```python
from build123d import *

# Parameters (mm, degrees)
BOSS_EXTRUDE1_DEPTH     = 10
CUT_EXTRUDE1_DEPTH      = 47.432747065
CUT_EXTRUDE1_DEPTH_BACK = 47.432747065
SKETCH2_R               = 1.65
CHAMFER1_SIZE           = 1.6
FILLET1_R               = 3
FILLET3_R               = 5


with BuildPart() as part:
    # Sketch1 → Boss-Extrude1 (new body)
    with BuildSketch(Plane.XY):
        Polygon((0, 0), (0, 5), (-13, 5), (-13, 25), (0, 25), (0, 30), (-34, 30), (-34, 25), (-21, 25), (-21, 5), (-34, 5), (-34, 0), align=None)
    extrude(amount=BOSS_EXTRUDE1_DEPTH)

    # Sketch2 → Cut-Extrude1 (cut, two sides: drawn at the far end of the back side and taken through both)
    with BuildSketch(Plane(origin=(0, 30, 0), x_dir=(1, 0, 0), z_dir=(0, 1, 0)).offset(-CUT_EXTRUDE1_DEPTH_BACK)):
        with Locations(Location((-30, -5, 0), (0, 0, 180))):
            Circle(SKETCH2_R)
        with Locations(Location((-4, -5, 0), (0, 0, 180))):
            Circle(SKETCH2_R)
    extrude(amount=CUT_EXTRUDE1_DEPTH + CUT_EXTRUDE1_DEPTH_BACK, mode=Mode.SUBTRACT)

    # Chamfer1
    chamfer1_edges = [part.edges().sort_by_distance(p)[0] for p in [
        (-28.35, 5, 5),
        (-2.35, 5, 5),
    ]]
    chamfer(chamfer1_edges, length=CHAMFER1_SIZE)

    # Fillet1
    fillet1_edges = [part.edges().sort_by_distance(p)[0] for p in [
        (-21, 5, 5),
        (-21, 25, 5),
        (-13, 25, 5),
        (-13, 5, 5),
    ]]
    fillet(fillet1_edges, radius=FILLET1_R)

    # Fillet3
    fillet3_edges = [part.edges().sort_by_distance(p)[0] for p in [
        (-34, 2.5, 0),
        (-34, 2.5, 10),
        (0, 2.5, 10),
        (0, 2.5, 0),
        (0, 27.5, 0),
        (0, 27.5, 10),
        (-34, 27.5, 0),
        (-34, 27.5, 10),
    ]]
    fillet(fillet3_edges, radius=FILLET3_R - 0.0001)  # a hair under: the kernel refuses the full size


solid = part.part
```
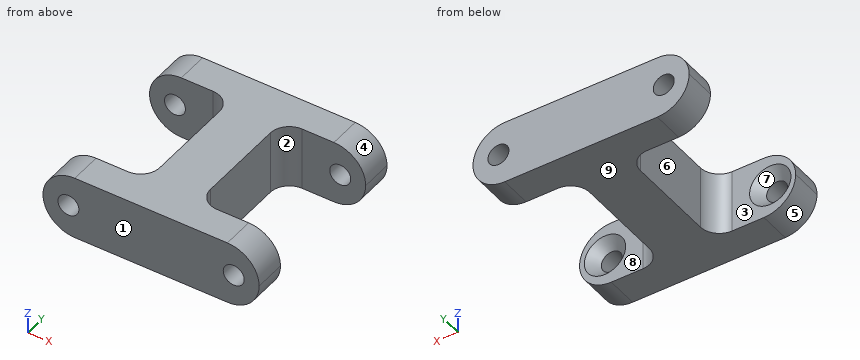
Geometry check sheet. Reference: the model listing, model coordinates, mm. Face numbers are marked on the shaded views. A direction names the side the tool comes from. Coordinates: 2 decimals unless noted, no trailing zeros. Order: outer loops, then holes, each group sorted by start corner. A loop starts at its lowest first (then second) coordinate and runs counter-clockwise, first axis right, second up. Notation, with made-up numbers: (-35.5, 88) - (8.5, 88) arc R26 cw to (8.5, 127) - close; hole circle Ø9 at (29, 89.5). An arc over 180 degrees is marked (long way). Answer as a JSON object with one key per item and string values. Group by question number.
Item 1: Sectioned sample at A-A, the plane x = -11.5. Record the cut outline in (y, z).
Item 2: Depth check by flat-ended pin: pin 1 Ø3 at (y, z) = (8, 2) entering from +X; pin 2 Ø6 at (y, z) = (11.5, 4) entering from +X; pin 3 Ø3 at (y, z) = (14, 6) entering from -X. Enter the tip coordinate at first touch or a pass-through.
Item 3: Sectioned sample at C-C, the plane z = 8.75. Record the cut outline in (x, y), and give its area (3 significant figures).
Item 4: Scan lines: probe 1 along X at (y, z) = (1.4, 5); probe 2 along Y at (x, z) = (-8, 7.75); probe 3 along X at (y, z) = (4, 6). Record each from-to range of solid material in increasing order.
Item 5: Tool access check on the marked faces 5, 6, 7, 8 and 9. Record the directions out of +Z, -Z, +X, -X, +Y, -Y that give a thin tool (end or side, any length) a straight path to the whole face; none if there is none.
Item 6: Sectioned sample at D-D, the plane x = -4. Record the cut outline in (y, z), and give its area (3 significant figures).
Item 7: Draft check along Y on the marked faces 1, 2, 3 and 4. Enter one of: +Y half, -Y half, draft (parallel to the pull), parting line (faces both ways), or undercut.
Item 8: Sectioned sample at B-B, the plane y = 20.75. Record the cut outline in (x, z), and give its area (3 significant figures).
Resolved:
{
 "1": {"outline": "(0, 0) - (5.4, 0) - (5.4, 10) - (0, 10) - close; (24.6, 0) - (30, 0) - (30, 10) - (24.6, 10) - close"},
 "2": {"pin 1": "x = -12.6", "pin 2": "x = -13", "pin 3": "x = -21"},
 "3": {"outline": "(-32.31, 0) - (-1.69, 0) - (-1.69, 5) - (-10, 5) arc R3 cw to (-13, 8) - (-13, 22) arc R3 cw to (-10, 25) - (-1.69, 25) - (-1.69, 30) - (-32.31, 30) - (-32.31, 25) - (-24, 25) arc R3 cw to (-21, 22) - (-21, 8) arc R3 cw to (-24, 5) - (-32.31, 5) - close", "area": "474 mm^2"},
 "4": {"probe 1": "-34 to -31.65, -28.35 to -5.65, -2.35 to 0", "probe 2": "0 to 5, 25 to 30", "probe 3": "-33.9 to -32.02, -27.98 to -6.02, -1.98 to -0.1"},
 "5": {"face 5": "-Z, -X, +Y, -Y", "face 6": "+Z, -Z, -X", "face 7": "none", "face 8": "+Z, -Z, +X", "face 9": "-Z, +X, -X, +Y, -Y"},
 "6": {"outline": "(0, 0.1) - (5, 0.1) - (5, 1.75) - (3.4, 3.35) - (0, 3.35) - close; (0, 6.65) - (3.4, 6.65) - (5, 8.25) - (5, 9.9) - (0, 9.9) - close; (25, 0.1) - (30, 0.1) - (30, 3.35) - (25, 3.35) - close; (25, 6.65) - (30, 6.65) - (30, 9.9) - (25, 9.9) - close", "area": "62.4 mm^2"},
 "7": {"face 1": "-Y half", "face 2": "undercut", "face 3": "undercut", "face 4": "draft"},
 "8": {"outline": "(-21, 0) - (-13, 0) - (-13, 10) - (-21, 10) - close", "area": "80.0 mm^2"}
}
